Design review of the part built by this model. Coordinates are the model's own, in mm. A direction names the side the tool comes from. Give positions to 0.01 mm unless a question says otherwise; leave off trailing zeros. Loops run counter-clockwise (first coordinate to the right, second up) from the corner with the lowest first, then second, coordinate; pieces in that order, holes last.
from build123d import *

# Parameters (mm, degrees)
BOSS_EXTRUDE1_DEPTH = 25.4
BOSS_EXTRUDE2_DEPTH = 9.525
BOSS_EXTRUDE3_START = 9.525
BOSS_EXTRUDE3_DEPTH = 9.525
CUT_EXTRUDE2_DEPTH  = 99.135296592
SKETCH6_W           = 12.7
SKETCH6_H           = 6.223
SKETCH6_H_2         = 6.35
CUT_EXTRUDE3_DEPTH  = 99.135296592


with BuildPart() as part:
    # Sketch1 → Boss-Extrude1 (new body)
    with BuildSketch(Plane.XY):
        with BuildLine():
            Line((-76.2, 0), (-81.713329641, -31.267646158))
            Line((-81.713329641, -31.267646158), (5.513329641, -31.267646158))
            Line((5.513329641, -31.267646158), (0, 0))
            ThreePointArc((0, 0), (-38.1, 10.208864232), (-76.2, 0))
        make_face()
    extrude(amount=BOSS_EXTRUDE1_DEPTH)

    # Sketch2 → Boss-Extrude2 (add)
    with BuildSketch(Plane.XY.offset(25.4)):
        with BuildLine():
            Line((-76.2, 12.7), (-76.2, 0))
            Line((-76.2, 0), (-81.713329641, -31.267646158))
            Line((-81.713329641, -31.267646158), (5.513329641, -31.267646158))
            Line((5.513329641, -31.267646158), (0, 0))
            Line((0, 0), (0, 12.7))
            ThreePointArc((0, 12.7), (-38.1, 29.898958349), (-76.2, 12.7))
        make_face()
    extrude(amount=BOSS_EXTRUDE2_DEPTH)

    # Sketch3 → Boss-Extrude3 (add)
    with BuildSketch(Plane(origin=(0, 0, 0), x_dir=(-1, 0, 0), z_dir=(0, 0, -1)).offset(BOSS_EXTRUDE3_START)):
        with BuildLine():
            Line((0, 0), (0, 12.7))
            ThreePointArc((0, 12.7), (38.1, 29.898958349), (76.2, 12.7))
            Line((76.2, 12.7), (76.2, 0))
            Line((76.2, 0), (81.713329641, -31.267646158))
            Line((81.713329641, -31.267646158), (-5.513329641, -31.267646158))
            Line((-5.513329641, -31.267646158), (0, 0))
        make_face()
    extrude(amount=-BOSS_EXTRUDE3_DEPTH)

    # Sketch5 → Cut-Extrude2 (cut, through all)
    with BuildSketch(Plane(origin=(0, 0, -9.525), x_dir=(-1, 0, 0), z_dir=(0, 0, -1))):
        with BuildLine():
            Line((-5.513329641, -31.267646158), (81.713329641, -31.267646158))
            ThreePointArc((81.713329641, -31.267646158), (38.1, -25.402967232), (-5.513329641, -31.267646158))
        make_face()
    extrude(amount=-CUT_EXTRUDE2_DEPTH, mode=Mode.SUBTRACT)

    # Sketch6 → Cut-Extrude3 (cut, through all)
    with BuildSketch(Plane(origin=(0, 0, -9.525), x_dir=(-1, 0, 0), z_dir=(0, 0, -1))):
        with Locations((13.536670359, -15.456146158)):
            Rectangle(SKETCH6_W, SKETCH6_H)
        with Locations((62.663329641, -15.392646158)):
            Rectangle(SKETCH6_W, SKETCH6_H_2)
    extrude(amount=-CUT_EXTRUDE3_DEPTH, mode=Mode.SUBTRACT)


solid = part.part
Q1. Take a section at B-B (x = -67). Give the boundary of the cut face in (y, z) (3 decimals), plus the area to 3 significant figures.
Results:
outline: (-27.952, -9.525) - (-18.568, -9.525) - (-18.568, 34.925) - (-27.952, 34.925) - close; (-12.218, -9.525) - (20.877, -9.525) - (20.877, 0) - (4.516, 0) - (4.516, 25.4) - (20.877, 25.4) - (20.877, 34.925) - (-12.218, 34.925) - close
area: 1,470 mm2
Q2. Wall thickness on line 1 (Z direction, x = -27, y = 17.5) (3 decimals); line 2 (X direction, y = -16.5, z = 26); line 3 (X direction, y = -13, z = -5): over which ranges is each line inside the solid? List them lowest first.
Results:
line 1: z = -9.525 to 0, 25.4 to 34.925
line 2: x = -79.11 to -69.01, -56.31 to -19.89, -7.19 to 2.91
line 3: x = -78.49 to -69.01, -56.31 to -19.89, -7.19 to 2.29
Q3. Take a section at C-C (y = -14.5). Give the boundary of the cut face in (x, z) (3 decimals).
Results:
outline: (-78.757, -9.525) - (-69.013, -9.525) - (-69.013, 34.925) - (-78.757, 34.925) - close; (-56.313, -9.525) - (-19.887, -9.525) - (-19.887, 34.925) - (-56.313, 34.925) - close; (-7.187, -9.525) - (2.557, -9.525) - (2.557, 34.925) - (-7.187, 34.925) - close
Q4. Draft analysis for pull direction Y (two halves, no side actions). For faces 1 (the face through (-37.541, 10.207, 12.522)), 2 (the face through (-56.313, -15, 12)), 3 (the face through (0, 6, -5)), state which applies: pulls with the +Y half, pulls with the -Y half, needs draft (parallel to the pull), parting line crosses it, or undercut.
Results:
face 1: pulls with the +Y half
face 2: undercut
face 3: needs draft
Q5. Take a section at D-D (y = -26.5). Give the boundary of the cut face in (x, z) (3 decimals).
Results:
outline: (-80.873, -9.525) - (-57.101, -9.525) - (-57.101, 34.925) - (-80.873, 34.925) - close; (-19.099, -9.525) - (4.673, -9.525) - (4.673, 34.925) - (-19.099, 34.925) - close
Q6. Insertion check: pin 1 (3 mm diameter, centred on y = 6, z = -5.5, fed in from +X); pin 2 (8 mm diameter, centred on x = -19, z = 17, fed in from +Y); pin 3 (7 mm diameter, centred on y = -15.5, z = 5, fed in from -X). Each pin has a flat end and moves straight along its axis. Give the tip position at first contact, or say it passes through.
Results:
pin 1: stops at x = 0
pin 2: stops at y = 8.7
pin 3: stops at x = -79.55
Q7. Tool access review of faces 4 (the face through (-19.887, -15, 12)), 5 (the face through (-39, 0, -9.525)), 6 (the face through (-76.2, 6, -5)), 7 (the face through (0, 6, 30)), 8 (the face through (-39, 0, 34.925)): name each direction out of +Z, -Z, +X, -X, +Y, -Y from which nothing blocks a thin tool from reaching the whole face with its end or side.
Results:
face 4: +Z, -Z
face 5: -Z, +X, -X, +Y, -Y
face 6: +Z, -Z, -X, +Y
face 7: +Z, -Z, +X, +Y
face 8: +Z, +X, -X, +Y, -Y
Q8. Take a section at A-A (z = 32). Give the boundary of the cut face in (x, y), plus the area to 3 significant figures.
Results:
outline: (-81.71, -31.27) arc R165.1 cw to (5.51, -31.27) - (0, 0) - (0, 12.7) arc R50.8 ccw to (-76.2, 12.7) - (-76.2, 0) - close; hole (-69.01, -18.57) - (-56.31, -18.57) - (-56.31, -12.22) - (-69.01, -12.22) - close; hole (-19.89, -18.57) - (-7.19, -18.57) - (-7.19, -12.34) - (-19.89, -12.34) - close
area: 3,930 mm2
